Check sheet for the modelled part. Datum: model origin and axes. Units: mm. Face numbers are marked on the shaded views. Give positions to 0.01 mm unless a question says otherwise; leave off trailing zeros. Loops run counter-clockwise (first coordinate to the right, second up) from the corner with the lowest first, then second, coordinate; pieces in that order, holes last. Notation, with made-up numbers: M 4.25,50.25 L 40.25,50.25 A22 cw 40.25,88.25 Z; hole C 54,-12.75 d8. An arc over 180 degrees is marked long. Write each question's results on one line, items separated by ' | '. Start each with the question number.
1. Sectioned sample at A-A on x = 0. Record the cut outline in (y, z), and give its area (3 significant figures).
2. Material ranges on line 1 along Z through (x, y) = (0, -16); line 2 along Z through (x, y) = (-4, -6.5); line 3 along Y through (x, z) = (-13, -56), recorded low to high.
3. Sectioned sample at B-B on y = -39.5. Record the cut outline in (x, z), and give its area (3 significant figures).
4. Draft check along X on the marked faces 1, 2, 3 and 4. Enter one of: pulls with the +X half, pulls with the -X half, needs draft (parallel to the pull), parting line crosses it, or undercut.
5. Sectioned sample at C-C on z = -114.5. Record the cut outline in (x, y), and give its area (3 significant figures).
6. Sectioned sample at D-D on y = -19.5. Record the cut outline in (x, z), and give its area (3 significant figures).
7. Go/stop test with flat-tipped pins: pin 1 (2 mm diameter, centred on x = 19.5, z = -16.5, fed in from -Y); pin 2 (2 mm diameter, centred on x = 0.5, y = -12.5, fed in from -Z); pin 3 (4 mm diameter, centred on x = 13, y = -24, fed in from +Z). Record where each tip stops, or that it passes through.
```python
from build123d import *

# Parameters (mm, degrees)
F0_R     = 12.7
F1_DEPTH = 25.4
F0_R_2   = 19.05
F2_DEPTH = 50.8


with BuildPart() as f1:
    # F0 (on Front) → F1 (new body)
    with BuildSketch(Plane.XZ):
        with BuildLine():
            ThreePointArc((-25.4, 0), (0, -25.4), (25.4, 0))
            ThreePointArc((25.4, 0), (0, 25.4), (-25.4, 0))
        make_face()
        Circle(F0_R, mode=Mode.SUBTRACT)
        with BuildLine():
            Line((36.909375, -91.3528319874), (25.4, 0))
            ThreePointArc((25.4, 0), (0, -25.4), (-25.4, 0))
            Line((-25.4, 0), (-36.909375, -91.3528319874))
            ThreePointArc((-36.909375, -91.3528319874), (0, -62.7031249516), (36.909375, -91.3528319874))
        make_face()
    extrude(amount=F1_DEPTH)

    # F0 (on Front) → F2 (join)
    with BuildSketch(Plane.XZ):
        with BuildLine():
            Line((38.1, -100.8031249516), (36.909375, -91.3528319874))
            ThreePointArc((36.909375, -91.3528319874), (0, -62.7031249516), (-36.909375, -91.3528319874))
            Line((-36.909375, -91.3528319874), (-38.1, -100.8031249516))
            ThreePointArc((-38.1, -100.8031249516), (0, -138.9031249516), (38.1, -100.8031249516))
        make_face()
        with Locations((0, -100.8031249516)):
            Circle(F0_R_2, mode=Mode.SUBTRACT)
    extrude(amount=F2_DEPTH)


solid = f1.part
```
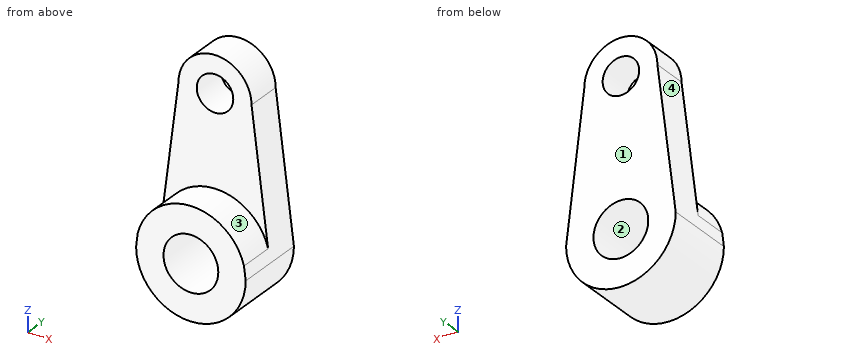
Output values:
1) outline: M -50.8,-138.9 L 0,-138.9 L 0,-119.85 L -50.8,-119.85 Z; M -50.8,-81.75 L 0,-81.75 L 0,-12.7 L -25.4,-12.7 L -25.4,-62.7 L -50.8,-62.7 Z; M -25.4,12.7 L 0,12.7 L 0,25.4 L -25.4,25.4 Z | area: 3,530 mm2
2) line 1: -138.9 to -119.85, -81.75 to -12.7, 12.7 to 25.4 | line 2: -138.69 to -119.43, -82.18 to -12.05, 12.05 to 25.08 | line 3: -25.4 to 0
3) outline: M -38.1,-100.8 A38.1 ccw 38.1,-100.8 L 36.91,-91.35 A38.1 ccw -36.91,-91.35 Z; hole C 0,-100.8 d38.1 | area: 3,420 mm2
4) face 1: needs draft | face 2: undercut | face 3: parting line crosses it | face 4: pulls with the -X half
5) outline: M -35.55,-50.8 L -13.24,-50.8 L -13.24,0 L -35.55,0 Z; M 13.24,-50.8 L 35.55,-50.8 L 35.55,0 L 13.24,0 Z | area: 2,270 mm2
6) outline: M -38.1,-100.8 A38.1 ccw 38.1,-100.8 L 25.4,0 A25.4 ccw -25.4,0 Z; hole C 0,-100.8 d38.1; hole C 0,0 d25.4 | area: 8,050 mm2
7) pin 1: y = -25.4 | pin 2: z = -138.9 | pin 3: z = 22.89
